Here's the drawing with two shaded views (mm, measured from the low corner). I have some questions. Give positions to 0.01 mm unless a question says otherwise; leave off trailing zeros.
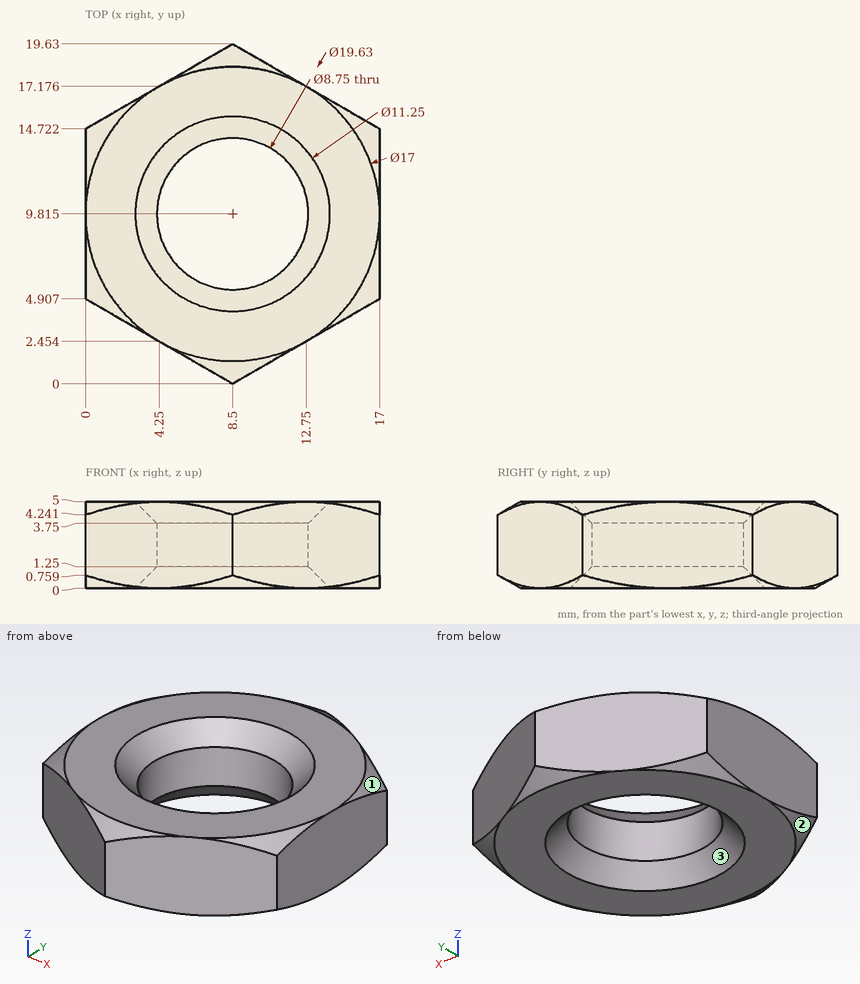
(1) Thinking about a two-plate mould opening in X: for the marked faces 1, 2 and 3, which applies, pulls with the +X half, pulls with the -X half, needs draft (parallel to the pull), parting line crosses it, or undercut?
Returned:
face 1: pulls with the +X half
face 2: pulls with the -X half
face 3: undercut
(2) Please list where these lines run through material, in increasing order: probe 1 along X at (y, z) = (6.5, 4.75) (1 decimal); probe 2 along Y at (x, z) = (7.75, 4.55) (1 decimal); probe 3 along X at (y, z) = (6, 0.75) (1 decimal).
Returned:
probe 1: x = 0.2 to 4.3, 12.7 to 16.8
probe 2: y = 0.6 to 4.7, 14.9 to 19.1
probe 3: x = 0 to 5.5, 11.5 to 17
(3) Will these pins go through, and if not, where does the flat tip stop? P1, Ø10, axis at x = 8.5, y = 5, coming from the +Z side; P2, Ø3, axis at x = 6, z = 1, coming from the -Y side.
Returned:
P1: stops at z = 5
P2: stops at y = 0.58
